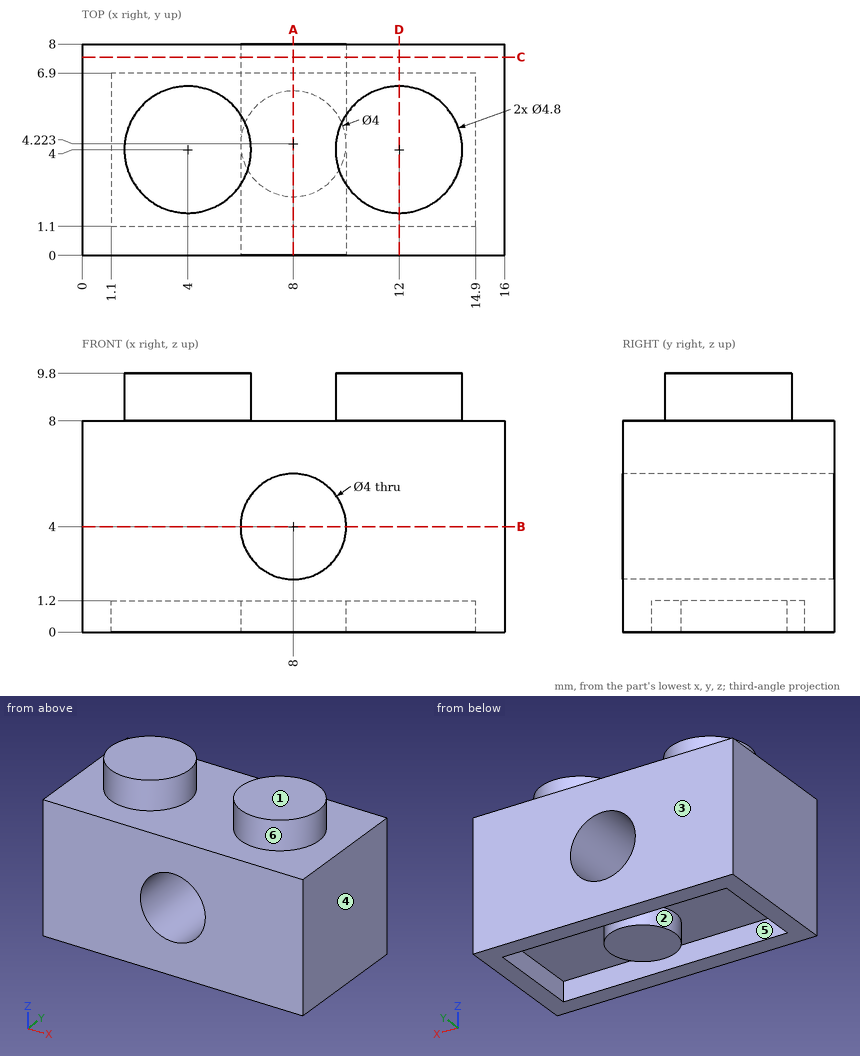
The figure shows three views and two pictorial views of one solid part (mm, origin at its lowest corner). Answer the questions. A direction names the side the tool comes from. Round coordinates to 2 decimals unless told otherwise and drop trailing zeros. Loops run counter-clockwise (first coordinate to the right, second up) from the corner with the lowest first, then second, coordinate; pieces in that order, holes last. Notation, with made-up numbers: M -29,-13.75 L -16,-13.75 A19 ccw -16,-7.75 Z; hole C -22.5,-32 d5. An arc over 180 degrees is marked long. Return JSON: item names as keys, results as strings.
Q1. Find section D-D, the plane x = 12. Determine the outline of the cut face in (y, z).
Results list:
{"outline": "M 0,0 L 1.1,0 L 1.1,1.2 L 6.9,1.2 L 6.9,0 L 8,0 L 8,8 L 6.4,8 L 6.4,9.8 L 1.6,9.8 L 1.6,8 L 0,8 Z"}
Q2. Find section A-A, the plane x = 8. Determine the outline of the cut face in (y, z).
Results list:
{"outline": "M 0,0 L 1.1,0 L 1.1,1.2 L 2.22,1.2 L 2.22,0 L 6.22,0 L 6.22,1.2 L 6.9,1.2 L 6.9,0 L 8,0 L 8,2 L 0,2 Z; M 0,6 L 8,6 L 8,8 L 0,8 Z"}
Q3. Which of the six approach directions +Z, -Z, +X, -X, +Y, -Y give full straight-line access (tool end or side, diameter ignored) to the marked faces 4, 5 and 6?
Results list:
{"face 4": "+Z, -Z, +X, +Y, -Y", "face 5": "-Z", "face 6": "+Z"}
Q4. Find section C-C, the plane y = 7.5. Determine the outline of the cut face in (x, z).
Results list:
{"outline": "M 0,0 L 16,0 L 16,8 L 0,8 Z; hole C 8,4 d4"}
Q5. The mould has two halves that part along Y. Classify the marked faces 1, 2 and 3: released by +Y, released by -Y, zero draft, split by the parting line, or undercut.
Results list:
{"face 1": "zero draft", "face 2": "undercut", "face 3": "released by +Y"}
Q6. This flat-tipped pin is pushed along its axis until it touches: pin 1 Ø1.5 at (x, y) = (4, 6) entering from -Z. Where does it stop, or does it pass through?
Results list:
{"pin 1": "stops at z = 1.2"}
Q7. Find the intervals of material crossed by line 1 along X through (y, z) = (2, 4); line 2 along Z through (x, y) = (8, 3); line 3 along X through (y, z) = (2.75, 4.5) (1 decimal), in increasing order. Write a range as from..to.
Results list:
{"line 1": "x = 0..6, 10..16", "line 2": "z = 0..2, 6..8", "line 3": "x = 0..6.1, 9.9..16"}
Q8. Find section B-B, the plane z = 4. Determine the outline of the cut face in (x, y).
Results list:
{"outline": "M 0,0 L 6,0 L 6,8 L 0,8 Z; M 10,0 L 16,0 L 16,8 L 10,8 Z"}
